```python
from build123d import *

# Parameters (mm, degrees)
SKETCH1_R           = 4
SKETCH1_R_2         = 3.075
BOSS_EXTRUDE1_DEPTH = 8
BOSS_EXTRUDE2_START = -5.5
SKETCH2_R           = 3.075
SKETCH2_R_2         = 1.5
BOSS_EXTRUDE2_DEPTH = 5.5
CHAMFER1_SIZE       = 0.2


with BuildPart() as part:
    # Sketch1 → Boss-Extrude1 (new body)
    with BuildSketch(Plane.XY):
        Circle(SKETCH1_R)
        Circle(SKETCH1_R_2, mode=Mode.SUBTRACT)
    extrude(amount=BOSS_EXTRUDE1_DEPTH)

    # Sketch2 → Boss-Extrude2 (add)
    with BuildSketch(Plane.XY.offset(8).offset(BOSS_EXTRUDE2_START)):
        Circle(SKETCH2_R)
        Circle(SKETCH2_R_2, mode=Mode.SUBTRACT)
    extrude(amount=BOSS_EXTRUDE2_DEPTH)

    # Chamfer1
    chamfer1_edges = [part.edges().sort_by_distance(p)[0] for p in [
        (-3.075, 0, 0),
    ]]
    chamfer(chamfer1_edges, length=CHAMFER1_SIZE)


solid = part.part
```
Could you check a few things on this model? Use its own coordinates, in mm. A direction names the side the tool comes from. Round coordinates to 2 decimals unless told otherwise and drop trailing zeros. Loops run counter-clockwise (first coordinate to the right, second up) from the corner with the lowest first, then second, coordinate; pieces in that order, holes last. Notation, with made-up numbers: (21.5, 63.25) - (69.5, 63.25) arc R25 cw to (69.5, 83.25) - close; hole circle Ø9 at (-39.5, -30). An arc over 180 degrees is marked (long way). Answer as CSV lines item,"result".
1. On a 3-axis mill with a long thin cutter (end or side, diameter ignored), from which of +Z, -Z, +X, -X, +Y, -Y can I reach the whole of each face in a straight line? I mean faces 1 (the face through (-0.67, -3, 1.33)), 2 (the face through (2, 0, 8)). Say none if no direction works.
Filled in:
face 1,"-Z"
face 2,"+Z, +X, -X, +Y, -Y"
2. I want a section at D-D on y = 3.5. List the corners of the cut face in (x, z) for me.
Filled in:
outline,"(-1.94, 0) - (1.94, 0) - (1.94, 8) - (-1.94, 8) - close"
3. I want a section at A-A on y = 0. List the corners of the cut face in (x, z) for me (3 decimals), then the cut area to 3 significant figures.
Filled in:
outline,"(-4, 0) - (-3.275, 0) - (-3.075, 0.2) - (-3.075, 2.5) - (-1.5, 2.5) - (-1.5, 8) - (-4, 8) - close; (1.5, 2.5) - (3.075, 2.5) - (3.075, 0.2) - (3.275, 0) - (4, 0) - (4, 8) - (1.5, 8) - close"
area,"32.1 mm^2"
4. We'd pull the mould along Y, two halves only. Please class faces 3 (the face through (-2, -3, 0)), 4 (the face through (-1.5, 0.07, 5.21)), 5 (the face through (-0.867, -3.905, 3.944)): +Y half, -Y half, draft (parallel to the pull), parting line (faces both ways), or undercut.
Filled in:
face 3,"draft"
face 4,"undercut"
face 5,"parting line"
5. I want a section at C-C on z = 3.25. List the corners of the cut face in (x, y) for me, then the cut area to 3 significant figures.
Filled in:
outline,"circle Ø8 at (0, 0); hole circle Ø3 at (0, 0)"
area,"43.2 mm^2"
6. Please list where these lines run through material, in increasing order: line 1 along Y through (x, z) = (0, 6.75); line 2 along Y through (x, z) = (0, 1.1) (3 decimals); line 3 along Z through (x, y) = (2, -1.25). Write a range as [from, to].
Filled in:
line 1,"y = [-4, -1.5], [1.5, 4]"
line 2,"y = [-4, -3.075], [3.075, 4]"
line 3,"z = [2.5, 8]"
7. For pin 1 Ø1.5 at (y, z) = (2, 6.5) entering from +X; pin 2 Ø4 at (x, y) = (-3, 3) entering from +Z; pin 3 Ø1 at (y, z) = (-2, 3) entering from -X; pin 4 Ø3 at (y, z) = (2.5, 3) entering from -X, each with a flat end and sliding along its axis, tell me the tip position at first contact or that it passes through.
Filled in:
pin 1,"stops at x = 3.8"
pin 2,"stops at z = 8"
pin 3,"stops at x = -3.71"
pin 4,"stops at x = -3.87"
